Design review of the part shown in the three views and the two pictorial views. Dimensions are in mm from the part's minimum x, y and z. A direction names the side the tool comes from. Round coordinates to 2 decimals unless told otherwise and drop trailing zeros. Order: outer loops, then holes, each group sorted by start corner. A loop starts at its lowest first (then second) coordinate and runs counter-clockwise, first axis right, second up.
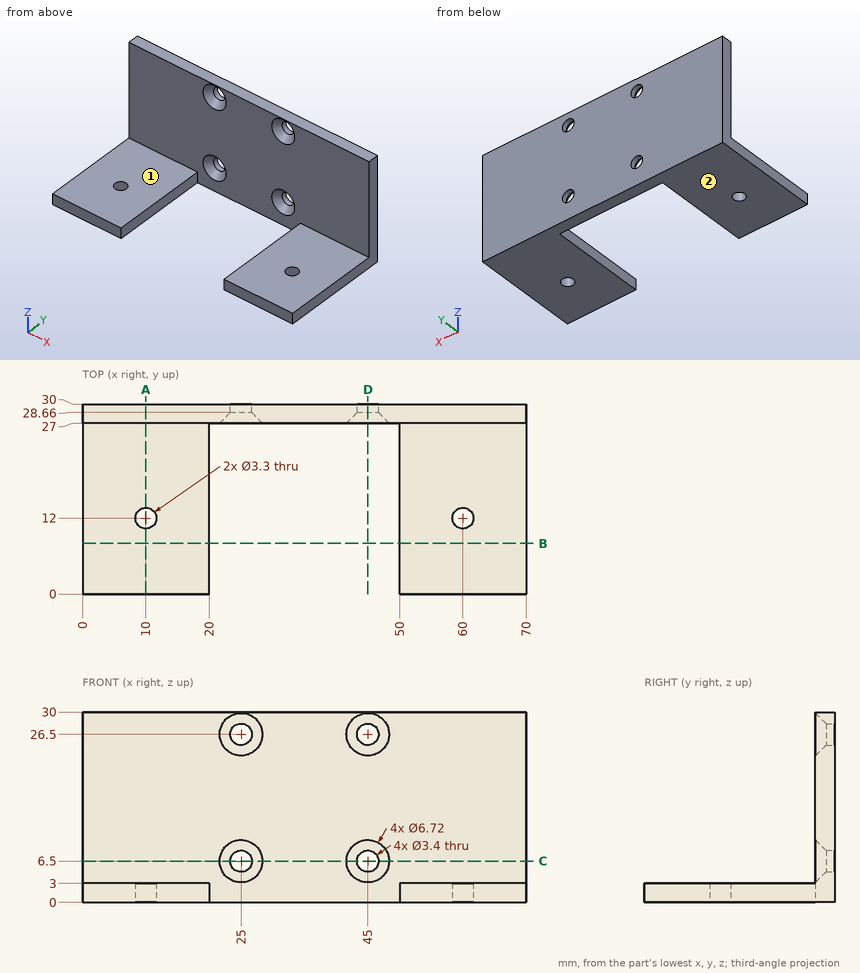
(1) Tool access review of the marked faces 1 and 2: name each direction out of +Z, -Z, +X, -X, +Y, -Y from which nothing blocks a thin tool from reaching the whole face with its end or side.
(2) Add section D-D on x = 45. Give the boundary of the cut face in (y, z).
(3) Clearance check with flat-ended pins moving along their axes: P1, Ø5, axis at x = 23, y = 9, coming from the +Z side; P2, Ø10, axis at x = 56, y = 17, coming from the +Z side; P3, Ø6, axis at x = 14, z = 19, coming from the -Y side; P4, Ø5.5, axis at x = 45, z = 6.5, coming from the -Y side. State where each tip first meets the part, or that it passes through.
(4) Add section C-C on z = 6.5. Give the boundary of the cut face in (x, y).
(5) Add section A-A on x = 10. Give the boundary of the cut face in (y, z).
(6) Wall thickness on L1, parallel to Z at x = 25, y = 29.5; L2, parallel to Y at x = 64.5, z = 9; L3, parallel to Y at x = 60, z = 1.2: over which ranges is each line inside the solid? List them lowest first.
(7) Add section B-B on y = 8. Give the boundary of the cut face in (x, z).
Here are the results:
1. face 1: +Z, +X, -X, -Y
1. face 2: -Z, +X, -X, +Y, -Y
2. outline: (27, 0) - (30, 0) - (30, 4.8) - (28.66, 4.8) - (27, 3.14) - close; (27, 9.86) - (28.66, 8.2) - (30, 8.2) - (30, 24.8) - (28.66, 24.8) - (27, 23.14) - close; (27, 29.86) - (28.66, 28.2) - (30, 28.2) - (30, 30) - (27, 30) - close
3. P1: passes through
3. P2: stops at z = 3
3. P3: stops at y = 27
3. P4: stops at y = 27.61
4. outline: (0, 27) - (21.64, 27) - (23.3, 28.66) - (23.3, 30) - (0, 30) - close; (26.7, 28.66) - (28.36, 27) - (41.64, 27) - (43.3, 28.66) - (43.3, 30) - (26.7, 30) - close; (46.7, 28.66) - (48.36, 27) - (70, 27) - (70, 30) - (46.7, 30) - close
5. outline: (0, 0) - (10.35, 0) - (10.35, 3) - (0, 3) - close; (13.65, 0) - (30, 0) - (30, 30) - (27, 30) - (27, 3) - (13.65, 3) - close
6. L1: z = 0 to 4.8, 8.2 to 24.8, 28.2 to 30
6. L2: y = 27 to 30
6. L3: y = 0 to 10.35, 13.65 to 30
7. outline: (0, 0) - (20, 0) - (20, 3) - (0, 3) - close; (50, 0) - (70, 0) - (70, 3) - (50, 3) - close
